Autodesk Inventor part; units mm, degrees
ref_plane "YZ Plane" through (0, 0, 0) normal (1, 0, 0) x (0, 1, 0)
ref_plane "XZ Plane" through (0, 0, 0) normal (0, 1, 0) x (-1, 0, 0)
ref_plane "XY Plane" through (0, 0, 0) normal (0, 0, 1) x (1, 0, 0)
sketch "草圖1" plane through (0, 0, 0) normal (0, 1, 0) x (-1, 0, 0)
  line L0 (0, 0) -> (100, 0)
  line L1 (100, 0) -> (100, -80)
  line L2 (100, -80) -> (0, -80)
  line L3 (0, -80) -> (0, 0)
  dimension "d0" = 100
  dimension "d1" = 80
extrude "擠出1" add sketch "草圖1" along normal blind 8
sketch "草圖2" plane through (0, 0, 0) normal (1, 0, 0) x (0, 0, -1)
  circle A0 centre (5, 4) radius 2.5
  line L0 (0, 0) -> (0, 8)
  line L1 (0, 8) -> (80, 8)
  point P0 (0, 4)
  dimension "d4" = 5
  dimension "d5" = 5
  dimension "d6" = 4
extrude "擠出2" cut sketch "草圖2" against normal blind 10
sketch "草圖3" plane through (-100, 0, -80) normal (-1, 0, 0) x (0, 0, 1)
  circle A0 centre (75, 4) radius 2.5
  circle A1 centre (75, 4) radius 2.5
  point P0 (80, 0)
extrude "擠出3" cut sketch "草圖3" against normal blind 10
sketch "草圖4" plane through (-100, 0, -80) normal (-1, 0, 0) x (0, 0, 1)
  point P0 (80, 0)
properties part number "MoneyCase_Lid"
For this review, take the finished solid that the model builds, in its own axes (mm). A direction names the side the tool comes from. Coordinates: 2 decimals unless noted, no trailing zeros. Loops run counter-clockwise (first coordinate to the right, second up) from the corner with the lowest first, then second, coordinate; pieces in that order, holes last. Notation, with made-up numbers: (77, -36) - (107, -36) arc R21 cw to (107, -16) - close; hole circle Ø7 at (35.25, 20). An arc over 180 degrees is marked (long way). Use a Markdown table: item, result. Add a question column.
Item 1: Tool access review of faces 5 (the face through (0, 4, -41)), 6 (the face through (-4.93, 4.751, -7.385)): name each direction out of +Z, -Z, +X, -X, +Y, -Y from which nothing blocks a thin tool from reaching the whole face with its end or side.
Item 2: For line 1 (Y direction, x = -7, z = -5); line 2 (Z direction, x = -6, y = 2); line 3 (Z direction, x = -3.5, y = 1.75), list the stretches that pass through material, from the lowest coordinate up.
Item 3: Mouldability with a two-part tool opening along Y and no side actions: class faces 1 (the face through (-49, 0, -39)), 2 (the face through (-90, 4, -5)), 3 (the face through (-95.07, 4.751, -2.615)), 4 (the face through (-100, 4, -39)) as pulls with the +Y half, pulls with the -Y half, needs draft (parallel to the pull), parting line crosses it, or undercut.
Item 4: We need section B-B (x = -94). Give the boundary of the cut face in (y, z), and give its area (3 significant figures).
Item 5: Insertion check: pin 1 Ø1.5 at (y, z) = (3, -5) entering from -X; pin 2 Ø4.5 at (y, z) = (4, -5) entering from +X. Each pin has a flat end and moves straight along its axis. Give the tip position at first contact, or say it passes through.
Item 6: We need section A-A (z = -5). Give the boundary of the cut face in (x, y).
Results list:
| question | item | result |
|---|---|---|
| 1 | face 5 | +Z, -Z, +X, +Y, -Y |
| 1 | face 6 | +X |
| 2 | line 1 | y = 0 to 1.5, 6.5 to 8 |
| 2 | line 2 | z = -80 to -6.5, -3.5 to 0 |
| 2 | line 3 | z = -80 to -6.09, -3.91 to 0 |
| 3 | face 1 | pulls with the -Y half |
| 3 | face 2 | undercut |
| 3 | face 3 | undercut |
| 3 | face 4 | needs draft |
| 4 | outline | (0, -80) - (8, -80) - (8, 0) - (0, 0) - close; hole circle Ø5 at (4, -5) |
| 4 | area | 620 mm^2 |
| 5 | pin 1 | stops at x = -90 |
| 5 | pin 2 | stops at x = -10 |
| 6 | outline | (-100, 0) - (0, 0) - (0, 1.5) - (-10, 1.5) - (-10, 6.5) - (0, 6.5) - (0, 8) - (-100, 8) - (-100, 6.5) - (-90, 6.5) - (-90, 1.5) - (-100, 1.5) - close |
